from build123d import *

# Parameters (mm, degrees)
ESQUISSE1_W             = 16
ESQUISSE1_H             = 12.5
ESQUISSE1_R             = 1.375
EXTRUSION1_DEPTH        = 1
EXTRUSION2_DEPTH        = 2
ENL_V_MAT_EXTRU_1_DEPTH = 2.25
CONG_1_R                = 0.02


with BuildPart() as part:
    # Esquisse1 → Extrusion1 (new body)
    with BuildSketch(Plane.XY):
        with Locations((-0.25, 0)):
            Rectangle(ESQUISSE1_W, ESQUISSE1_H)
        with Locations((0.75, 4.15)):
            Circle(ESQUISSE1_R, mode=Mode.SUBTRACT)
    extrude(amount=EXTRUSION1_DEPTH)

    # Esquisse3 → Extrusion2 (add)
    with BuildSketch(Plane.XY):
        Polygon((1.5, -1), (5, -1), (5, -3.25), (4.5, -3.75), (1.5, -3.75), align=None)
    extrude(amount=EXTRUSION2_DEPTH)

    # Esquisse4 → Enlèv. mat.-Extru.1 (cut)
    with BuildSketch(Plane.XZ.offset(3.5)):
        with BuildLine():
            Line((1.905461948, 2), (2.855665367, 2))
            ThreePointArc((2.855665367, 2), (2.380563657, 1.872882694), (1.905461948, 2))
        make_face()
        with BuildLine():
            Line((4.463762682, 2), (3.513559263, 2))
            ThreePointArc((3.513559263, 2), (3.988660973, 1.872882694), (4.463762682, 2))
        make_face()
    extrude(amount=-ENL_V_MAT_EXTRU_1_DEPTH, mode=Mode.SUBTRACT)

    # Congé1
    cong_1_edges = [part.edges().sort_by_distance(p)[0] for p in [
        (3.25, -1, 2),
        (5, -2.125, 2),
        (4.75, -3.5, 2),
        (3, -3.75, 2),
        (1.5, -2.375, 2),
        (3.988660973, -3.5, 2),
        (3.513559263, -2.375, 2),
        (3.988660973, -1.25, 2),
        (4.463762682, -2.375, 2),
        (1.905461948, -2.375, 2),
        (2.380563657, -1.25, 2),
        (2.855665367, -2.375, 2),
        (2.380563657, -3.5, 2),
    ]]
    fillet(cong_1_edges, radius=CONG_1_R)


solid = part.part
Can you work these out from the model? Positions are in its coordinate system, mm. A direction names the side the tool comes from. Round coordinates to 2 decimals unless told otherwise and drop trailing zeros. Write each loop counter-clockwise with the first axis right and the second up, starting at its lowest first coordinate (ties: lowest second). Pieces come first, ordered by that corner, then holes. Notation, with made-up numbers: M 14.25,8 L 61.25,8 A24 ccw 61.25,19 Z; hole C 81.25,-29 d11. An arc over 180 degrees is marked long. Use CSV: the item, a comma, the result in double quotes.
(1) I'm going to push flat-ended pins straight in: pin 1 (1.5 mm diameter, centred on x = 1, y = 0, fed in from +Z); pin 2 (0.8 mm diameter, centred on x = 3.5, z = 1.5, fed in from -Y); pin 3 (0.5 mm diameter, centred on y = -2, z = 1.5, fed in from +X). Where does each tip first touch, or does it pass through?
Check values:
pin 1,"z = 1"
pin 2,"y = -3.75"
pin 3,"x = 5"
(2) On a 3-axis mill with a long thin cutter (end or side, diameter ignored), from which of +Z, -Z, +X, -X, +Y, -Y can I reach the whole of each face in a straight line? I mean faces 1 (the flat face through (3, -3.75, 1.5)), 2 (the cylindrical face through (3.982, -2.391, 1.873)), 3 (the flat face through (1.5, -2.4, 1.5)), 4 (the flat face through (3.2, -1, 1.5)). Say none if no direction works.
Check values:
face 1,"+Z, +X, -X, -Y"
face 2,"+Z"
face 3,"+Z, -X, +Y, -Y"
face 4,"+Z, +X, -X, +Y"
(3) Imagine slicing it at B-B (y = 4.15). Write out the boundary of the cut face in (x, z) (3 decimals).
Check values:
outline,"M -8.25,0 L -0.625,0 L -0.625,1 L -8.25,1 Z; M 2.125,0 L 7.75,0 L 7.75,1 L 2.125,1 Z"
(4) I need wall thicknesses on line 1 along Y through (x, z) = (0.75, 0.6) (3 decimals); line 2 along Z through (x, y) = (1.75, 0.25); line 3 along X through (y, z) = (3.5, 0.25). Which ranges of each line are inside material? Lowest first, please.
Check values:
line 1,"-6.25 to 2.775, 5.525 to 6.25"
line 2,"0 to 1"
line 3,"-8.25 to -0.46, 1.96 to 7.75"
(5) Imagine slicing it at C-C (z = 0.65). Write out the boundary of the cut face in (x, y) (3 decimals).
Check values:
outline,"M -8.25,-6.25 L 7.75,-6.25 L 7.75,6.25 L -8.25,6.25 Z; hole C 0.75,4.15 d2.75"
(6) Imagine slicing it at A-A (x = 0.75). Write out the boundary of the cut face in (y, z) (3 decimals), plus the area to 3 significant figures.
Check values:
outline,"M -6.25,0 L 2.775,0 L 2.775,1 L -6.25,1 Z; M 5.525,0 L 6.25,0 L 6.25,1 L 5.525,1 Z"
area,"9.75 mm^2"
(7) We'd pull the mould along Y, two halves only. Please class faces 5 (the cylindrical face through (0.45, 2.81, 0.49)), 6 (the flat face through (-0.4, 6.25, 0.5)), 7 (the flat face through (7.75, -0.1, 0.5)): +Y half, -Y half, draft (parallel to the pull), parting line (faces both ways), or undercut.
Check values:
face 5,"undercut"
face 6,"+Y half"
face 7,"draft"
